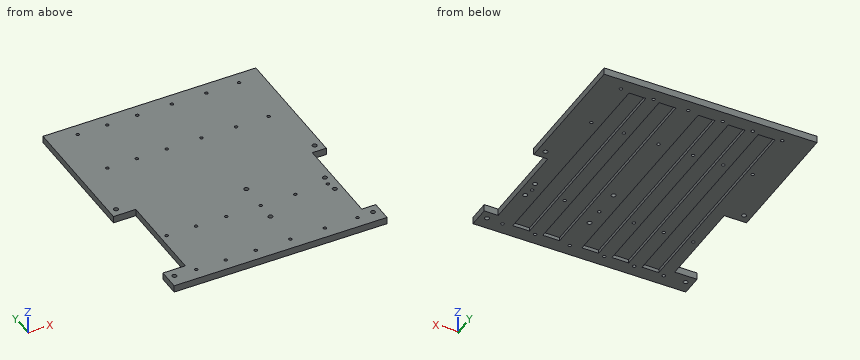
```python
from build123d import *

# Parameters (mm, degrees)
SKETCH_R             = 1.6
PAD_DEPTH            = 5
PAD_FACE8_W          = 152.4
PAD_FACE8_H          = 5
PAD001_DEPTH         = 80
SKETCH001_W          = 12
SKETCH001_H          = 156.9
POCKET_DEPTH         = 2.5
SKETCH002_W          = 12
SKETCH002_H          = 156.9
POCKET001_DEPTH      = 2.5
SKETCH003_W          = 12
SKETCH003_H          = 156.9
POCKET002_DEPTH      = 2.5
SKETCH004_W          = 12
SKETCH004_H          = 156.9
POCKET003_DEPTH      = 2.5
SKETCH005_W          = 12
SKETCH005_H          = 156.9
POCKET004_DEPTH      = 2.5
SKETCH006_R          = 1.1303
POCKET005_DEPTH      = 5.001
POCKET005_DEPTH_BACK = 0.001


with BuildPart() as part:
    # Sketch (on Face12378 of Binder) → Pad (new body)
    with BuildSketch(Plane(origin=(0, 0, 0), x_dir=(1, 0, 0), z_dir=(0, 0, -1))):
        Polygon((76.275, 138.125), (228.675, 138.125), (228.675, 122.9688), (218.675, 122.9688), (218.675, 56.2288), (228.675, 56.2288), (228.675, 41.225), (76.275, 41.225), (76.275, 56.2288), (92.275, 56.2288), (92.275, 122.9688), (76.275, 122.9688), align=None)
        with Locations((81.2788, 128.9688)):
            Circle(SKETCH_R, mode=Mode.SUBTRACT)
        with Locations((223.5188, 128.9688)):
            Circle(SKETCH_R, mode=Mode.SUBTRACT)
        with Locations((223.5188, 50.2288)):
            Circle(SKETCH_R, mode=Mode.SUBTRACT)
        with Locations((81.2788, 50.2288)):
            Circle(SKETCH_R, mode=Mode.SUBTRACT)
        with Locations((164, 102.75)):
            Circle(SKETCH_R, mode=Mode.SUBTRACT)
        with Locations((164, 70.25)):
            Circle(SKETCH_R, mode=Mode.SUBTRACT)
        with Locations((213.5, 83)):
            Circle(SKETCH_R, mode=Mode.SUBTRACT)
        with Locations((213.5188, 96.2288)):
            Circle(SKETCH_R, mode=Mode.SUBTRACT)
    extrude(amount=PAD_DEPTH)

    # Pad Face8 → Pad001 (add)
    with BuildSketch(Plane(origin=(152.475, -41.225, -2.5), x_dir=(1, 0, 0), z_dir=(0, 1, 0))):
        Rectangle(PAD_FACE8_W, PAD_FACE8_H)
    extrude(amount=PAD001_DEPTH)

    # Sketch001 (on Face23 of Pad001) → Pocket (cut)
    with BuildSketch(Plane(origin=(0, 0, -5), x_dir=(1, 0, 0), z_dir=(0, 0, -1))):
        with Locations((199.5188, 49.675)):
            Rectangle(SKETCH001_W, SKETCH001_H)
    extrude(amount=-POCKET_DEPTH, mode=Mode.SUBTRACT)

    # Sketch002 (on Face23 of Pocket) → Pocket001 (cut)
    with BuildSketch(Plane(origin=(0, 0, -5), x_dir=(1, 0, 0), z_dir=(0, 0, -1))):
        with Locations((178, 49.675)):
            Rectangle(SKETCH002_W, SKETCH002_H)
    extrude(amount=-POCKET001_DEPTH, mode=Mode.SUBTRACT)

    # Sketch003 (on Face5 of Pocket001) → Pocket002 (cut)
    with BuildSketch(Plane(origin=(0, 0, -5), x_dir=(1, 0, 0), z_dir=(0, 0, -1))):
        with Locations((150, 49.675)):
            Rectangle(SKETCH003_W, SKETCH003_H)
    extrude(amount=-POCKET002_DEPTH, mode=Mode.SUBTRACT)

    # Sketch004 (on Face5 of Pocket002) → Pocket003 (cut)
    with BuildSketch(Plane(origin=(0, 0, -5), x_dir=(1, 0, 0), z_dir=(0, 0, -1))):
        with Locations((128.4812, 49.675)):
            Rectangle(SKETCH004_W, SKETCH004_H)
    extrude(amount=-POCKET003_DEPTH, mode=Mode.SUBTRACT)

    # Sketch005 (on Face5 of Pocket003) → Pocket004 (cut)
    with BuildSketch(Plane(origin=(0, 0, -5), x_dir=(1, 0, 0), z_dir=(0, 0, -1))):
        with Locations((106.9624, 49.675)):
            Rectangle(SKETCH005_W, SKETCH005_H)
    extrude(amount=-POCKET004_DEPTH, mode=Mode.SUBTRACT)

    # Sketch006 (on Face5 of Pocket004) → Pocket005 (cut, two sides)
    with BuildSketch(Plane(origin=(0, 0, -5), x_dir=(1, 0, 0), z_dir=(0, 0, -1))) as pocket005_sk:
        with Locations((212.0969, 129.5538)):
            Circle(SKETCH006_R)
        with Locations((212.0969, 89.6144)):
            Circle(SKETCH006_R)
        with Locations((212.0969, 89.6144)):
            Circle(SKETCH006_R)
        with Locations((212.0969, 9.7356)):
            Circle(SKETCH006_R)
        with Locations((212.0969, -30.2038)):
            Circle(SKETCH006_R)
        with Locations((164, 89.6144)):
            Circle(SKETCH006_R)
        with Locations((188.7594, 89.6144)):
            Circle(SKETCH006_R)
        with Locations((139.2406, 89.6144)):
            Circle(SKETCH006_R)
        with Locations((117.7218, 89.6144)):
            Circle(SKETCH006_R)
        with Locations((96.6187, 89.6144)):
            Circle(SKETCH006_R)
        with Locations((96.6187, 129.5538)):
            Circle(SKETCH006_R)
        with Locations((117.7218, 129.5538)):
            Circle(SKETCH006_R)
        with Locations((139.2406, 129.5538)):
            Circle(SKETCH006_R)
        with Locations((164, 129.5538)):
            Circle(SKETCH006_R)
        with Locations((188.7594, 129.5538)):
            Circle(SKETCH006_R)
        with Locations((96.6187, 89.6144)):
            Circle(SKETCH006_R)
        with Locations((117.7218, 89.6144)):
            Circle(SKETCH006_R)
        with Locations((139.2406, 89.6144)):
            Circle(SKETCH006_R)
        with Locations((164, 89.6144)):
            Circle(SKETCH006_R)
        with Locations((188.7594, 89.6144)):
            Circle(SKETCH006_R)
        with Locations((164, 9.7356)):
            Circle(SKETCH006_R)
        with Locations((139.2406, 9.7356)):
            Circle(SKETCH006_R)
        with Locations((117.7218, 9.7356)):
            Circle(SKETCH006_R)
        with Locations((96.6187, 9.7356)):
            Circle(SKETCH006_R)
        with Locations((96.6187, -30.2038)):
            Circle(SKETCH006_R)
        with Locations((117.7218, -30.2038)):
            Circle(SKETCH006_R)
        with Locations((139.2406, -30.2038)):
            Circle(SKETCH006_R)
        with Locations((164, -30.2038)):
            Circle(SKETCH006_R)
        with Locations((188.7594, -30.2038)):
            Circle(SKETCH006_R)
        with Locations((188.7594, 9.7356)):
            Circle(SKETCH006_R)
    extrude(amount=-POCKET005_DEPTH, mode=Mode.SUBTRACT)
    extrude(pocket005_sk.sketch, amount=POCKET005_DEPTH_BACK, mode=Mode.SUBTRACT)


solid = part.part
```
The listing builds one solid part. Answer for the finished solid, in the listing's coordinates (mm). Give positions to 0.01 mm unless a question says otherwise; leave off trailing zeros. Order: outer loops, then holes, each group sorted by start corner. A loop starts at its lowest first (then second) coordinate and runs counter-clockwise, first axis right, second up. Notation, with made-up numbers: (63, 76) - (90, 76) arc R26 cw to (90, 106) - close; hole circle Ø4 at (59, 64). An arc over 180 degrees is marked (long way). Use one line per item in the form item = value. Start each with the question number.
(1) Consider line 1 (X direction, y = -73.5, z = -2.85) (3 decimals); line 2 (X direction, y = -24, z = -4.5) (3 decimals); line 3 (Y direction, x = 87, z = -1.45) (3 decimals). Determine where each line is inside the solid, lowest interval first. Write a range as from..to.
(2) A cutting plane is placed at B-B, the plane y = 13. Write down the section's boundary in (x, z) (3 decimals).
(3) Flat-ended cylindrical pins translate along their axes: pin 1 Ø2 at (y, z) = (-67, -4) entering from +X (3 decimals); pin 2 Ø1.5 at (x, y) = (198.5, -1) entering from -Z. Find the tip coordinate at first contact, or state that the pin passes through.
(4) A cutting plane is placed at C-C, the plane z = -3.8. State how many separate pieces and enclosed holes the cut face has, then the cut area to 3 significant figures.
(5) A cutting plane is placed at A-A, the plane x = 88. Write down the section's boundary in (y, z) (3 decimals).
Ans:
q1.line_1 = 92.275..100.962, 112.962..122.481, 134.481..144, 156..172, 184..193.519, 205.519..218.675
q1.line_2 = 76.275..100.962, 112.962..122.481, 134.481..144, 156..172, 184..193.519, 205.519..228.675
q1.line_3 = -138.125..-122.969, -56.229..38.775
q2.outline = (76.275, -5) - (100.962, -5) - (100.962, -2.5) - (112.962, -2.5) - (112.962, -5) - (122.481, -5) - (122.481, -2.5) - (134.481, -2.5) - (134.481, -5) - (144, -5) - (144, -2.5) - (156, -2.5) - (156, -5) - (172, -5) - (172, -2.5) - (184, -2.5) - (184, -5) - (193.519, -5) - (193.519, -2.5) - (205.519, -2.5) - (205.519, -5) - (228.675, -5) - (228.675, 0) - (76.275, 0) - close
q3.pin_1 = 218.675
q3.pin_2 = -2.5
q4.separate_pieces = 1
q4.enclosed_holes = 37
q4.area = 15,600 mm^2
q5.outline = (-138.125, -5) - (-122.969, -5) - (-122.969, 0) - (-138.125, 0) - close; (-56.229, -5) - (38.775, -5) - (38.775, 0) - (-56.229, 0) - close
